```python
from build123d import *

# Parameters (mm, degrees)
SKETCH1_W           = 12
SKETCH1_H           = 20
SKETCH1_W_2         = 10
SKETCH1_H_2         = 18
BOSS_EXTRUDE1_DEPTH = 400
SKETCH2_R           = 1.5
CUT_EXTRUDE1_DEPTH  = 200


with BuildPart() as part:
    # Sketch1 → Boss-Extrude1 (new body)
    with BuildSketch(Plane.XY):
        Rectangle(SKETCH1_W, SKETCH1_H)
        Rectangle(SKETCH1_W_2, SKETCH1_H_2, mode=Mode.SUBTRACT)
    extrude(amount=BOSS_EXTRUDE1_DEPTH)

    # Sketch2 → Cut-Extrude1 (cut)
    with BuildSketch(Plane(origin=(6, 0, 0), x_dir=(0, 0, -1), z_dir=(1, 0, 0))):
        with Locations(Location((-200, 0, 0), (0, 0, 90))):
            Circle(SKETCH2_R)
        with Locations(Location((-182, 0, 0), (0, 0, 90))):
            Circle(SKETCH2_R)
        with Locations(Location((-218, 0, 0), (0, 0, 90))):
            Circle(SKETCH2_R)
        with Locations(Location((-370, 0, 0), (0, 0, 90))):
            Circle(SKETCH2_R)
        with Locations(Location((-388, 0, 0), (0, 0, 90))):
            Circle(SKETCH2_R)
        with Locations(Location((-352, 0, 0), (0, 0, 90))):
            Circle(SKETCH2_R)
    extrude(amount=-CUT_EXTRUDE1_DEPTH, mode=Mode.SUBTRACT)


solid = part.part
```
Part model, mm, in its own coordinate system. A direction names the side the tool comes from. Give positions to 0.01 mm unless a question says otherwise; leave off trailing zeros. Order: outer loops, then holes, each group sorted by start corner. A loop starts at its lowest first (then second) coordinate and runs counter-clockwise, first axis right, second up. Notation, with made-up numbers: M 1.25,83 L 10.25,83 A13 cw 10.25,96 Z; hole C 23,61.25 d10. An arc over 180 degrees is marked long. Use a Markdown table: item, result. Add a question column.
(1) Drop a flat-ended pin along its axis: P1, Ø1.8, axis at y = 0, z = 388, coming from the +X side. Give the stop position or say it passes through.
(2) Saw through at C-C, the plane z = 127.5. Give the cut face in (x, y), and give its area (3 significant figures).
(3) Mould opens along Y. For faces 1 (the face through (0, 10, 197)), 2 (the face through (-5, 0, 197)), 3 (the face through (0, -10, 197)), 4 (the face through (0, 9, 197)) say: +Y half, -Y half, draft (parallel to the pull), parting line (faces both ways), or undercut.
(4) Saw through at A-A, the plane x = -2.25. Give the cut face in (y, z), and give its area (3 significant figures).
(5) Saw through at B-B, the plane y = 5.5. Give the cut face in (x, z).
(6) 3-axis set-ups, long thin cutter, end or side, ignore diameter. For faces 5 (the face through (-5.4, 0.8, 400)), 6 (the face through (0, -9, 197)): which of +Z, -Z, +X, -X, +Y, -Y reach the whole face in a straight line?
(7) Probe line 1 along X through (y, z) = (4.25, 350); line 2 along Y through (x, z) = (5.2, 218); line 3 along Y through (x, z) = (0.5, 359). List the from-to ranges inside material, lowest first. Write a range as [from, to].
Answer key:
| question | item | result |
|---|---|---|
| 1 | P1 | through |
| 2 | outline | M -6,-10 L 6,-10 L 6,10 L -6,10 Z; hole M -5,-9 L 5,-9 L 5,9 L -5,9 Z |
| 2 | area | 60.0 mm^2 |
| 3 | face 1 | +Y half |
| 3 | face 2 | undercut |
| 3 | face 3 | -Y half |
| 3 | face 4 | undercut |
| 4 | outline | M -10,0 L -9,0 L -9,400 L -10,400 Z; M 9,0 L 10,0 L 10,400 L 9,400 Z |
| 4 | area | 800 mm^2 |
| 5 | outline | M -6,0 L -5,0 L -5,400 L -6,400 Z; M 5,0 L 6,0 L 6,400 L 5,400 Z |
| 6 | face 5 | +Z, +X, -X, +Y, -Y |
| 6 | face 6 | +Z, -Z |
| 7 | line 1 | [-6, -5], [5, 6] |
| 7 | line 2 | [-10, -1.5], [1.5, 10] |
| 7 | line 3 | [-10, -9], [9, 10] |
